from build123d import *

# Parameters (mm, degrees)
SKETCH1_W           = 55
SKETCH1_H           = 55
BOSS_EXTRUDE1_DEPTH = 327.5
SKETCH2_R           = 22.5
CUT_EXTRUDE1_DEPTH  = 55
CUT_EXTRUDE2_DEPTH  = 55
SKETCH4_W           = 45
SKETCH4_H           = 45
CUT_EXTRUDE3_DEPTH  = 280


with BuildPart() as part:
    # Sketch1 → Boss-Extrude1 (new body)
    with BuildSketch(Plane.XY):
        Rectangle(SKETCH1_W, SKETCH1_H)
    extrude(amount=BOSS_EXTRUDE1_DEPTH)

    # Sketch2 → Cut-Extrude1 (cut)
    with BuildSketch(Plane(origin=(27.5, 0, 0), x_dir=(0, 0, -1), z_dir=(1, 0, 0))):
        with Locations((-27.5, 0)):
            Circle(SKETCH2_R)
    extrude(amount=-CUT_EXTRUDE1_DEPTH, mode=Mode.SUBTRACT)

    # Sketch3 → Cut-Extrude2 (cut)
    with BuildSketch(Plane(origin=(27.5, 0, 0), x_dir=(0, 0, -1), z_dir=(1, 0, 0))):
        with BuildLine():
            Line((0, 27.5), (-27.5, 27.5))
            ThreePointArc((-27.5, 27.5), (-8.054563517, 19.445436483), (0, 0))
            Line((0, 0), (0, 27.5))
        make_face()
        with BuildLine():
            Line((0, -27.5), (0, 0))
            ThreePointArc((0, 0), (-8.054563517, -19.445436483), (-27.5, -27.5))
            Line((-27.5, -27.5), (0, -27.5))
        make_face()
    extrude(amount=-CUT_EXTRUDE2_DEPTH, mode=Mode.SUBTRACT)

    # Sketch4 → Cut-Extrude3 (cut)
    with BuildSketch(Plane.XY.offset(327.5)):
        Rectangle(SKETCH4_W, SKETCH4_H)
    extrude(amount=-CUT_EXTRUDE3_DEPTH, mode=Mode.SUBTRACT)


solid = part.part
Design review of the part built by this model. Coordinates are the model's own, in mm. A direction names the side the tool comes from. Round coordinates to 2 decimals unless told otherwise and drop trailing zeros. Loops run counter-clockwise (first coordinate to the right, second up) from the corner with the lowest first, then second, coordinate; pieces in that order, holes last. Notation, with made-up numbers: M 79.5,16.25 L 91.5,16.25 A17 cw 91.5,22.25 Z; hole C 0,46 d9. An arc over 180 degrees is marked long. Answer as a JSON object with one key per item and string values.
Item 1: We need section B-B on z = 290. Give the boundary of the cut face in (x, y).
Answer sheet:
{"outline": "M -27.5,-27.5 L 27.5,-27.5 L 27.5,27.5 L -27.5,27.5 Z; hole M -22.5,-22.5 L 22.5,-22.5 L 22.5,22.5 L -22.5,22.5 Z"}
Item 2: We need section D-D on y = 4.5. Give the boundary of the cut face in (x, z), and give its area (3 significant figures).
Answer sheet:
{"outline": "M -27.5,0.37 L 27.5,0.37 L 27.5,5.45 L -27.5,5.45 Z; M -27.5,49.55 L -22.5,49.55 L -22.5,327.5 L -27.5,327.5 Z; M 22.5,49.55 L 27.5,49.55 L 27.5,327.5 L 22.5,327.5 Z", "area": "3,060 mm^2"}
Item 3: We need section C-C on x = 4. Give the boundary of the cut face in (y, z), and give its area (3 significant figures).
Answer sheet:
{"outline": "M -27.5,27.5 A27.5 ccw 27.5,27.5 L 27.5,327.5 L 22.5,327.5 L 22.5,47.5 L 10.31,47.5 A22.5 cw long -10.31,47.5 L -22.5,47.5 L -22.5,327.5 L -27.5,327.5 Z", "area": "3,530 mm^2"}
Item 4: Wall thickness on L1, parallel to X at y = 16.5, z = 181; L2, parallel to Z at x = 9, y = 0: over which ranges is each line inside the solid? List them lowest first. Write a range as from..to.
Answer sheet:
{"L1": "x = -27.5..-22.5, 22.5..27.5", "L2": "z = 0..5"}
Item 5: We need section A-A on y = -14. Give the boundary of the cut face in (x, z).
Answer sheet:
{"outline": "M -27.5,3.83 L 27.5,3.83 L 27.5,9.89 L -27.5,9.89 Z; M -27.5,45.11 L 27.5,45.11 L 27.5,327.5 L 22.5,327.5 L 22.5,47.5 L -22.5,47.5 L -22.5,327.5 L -27.5,327.5 Z"}
Item 6: Clearance check with flat-ended pins moving along their axes: P1, Ø12, axis at x = -7.5, y = -19.5, coming from the -Z side; P2, Ø10, axis at x = 6.5, y = 13.5, coming from the +Z side. State where each tip first meets the part, or that it passes through.
Answer sheet:
{"P1": "stops at z = 3.54", "P2": "stops at z = 47.5"}
Item 7: Machinability: for faces 4 (the flat face through (0, -22.5, 189)), 5 (the flat face through (-25, 0, 327.5)), which of the approach directions +Z, -Z, +X, -X, +Y, -Y give a long, thin tool a straight path to every point of the face, cutting with its end or side? Answer none if there is none.
Answer sheet:
{"face 4": "+Z", "face 5": "+Z, +X, -X, +Y, -Y"}
Item 8: The part is to be moulded in two halves that separate along X. For faces 1 (the flat face through (0, -27.5, 175)), 2 (the flat face through (0, 16, 47.5)), 3 (the flat face through (27.5, 0, 161)), say which applies: pulls with the +X half, pulls with the -X half, needs draft (parallel to the pull), parting line crosses it, or undercut.
Answer sheet:
{"face 1": "needs draft", "face 2": "undercut", "face 3": "pulls with the +X half"}
